from build123d import *

# Parameters (mm, degrees)
F0_R     = 33
F1_DEPTH = 10
F2_R     = 31.5
F3_DEPTH = 8
F5_DEPTH = 1
F6_R     = 1


with BuildPart() as f1:
    # F0 (on Top) → F1 (new body)
    with BuildSketch(Plane.XY):
        Circle(F0_R)
    extrude(amount=F1_DEPTH)

    # F2 (on face) → F3 (cut)
    with BuildSketch(Plane(origin=(0, 0, 0), x_dir=(1, 0, 0), z_dir=(0, 0, -1))):
        Circle(F2_R)
    extrude(amount=-F3_DEPTH, mode=Mode.SUBTRACT)

    # F4 (on face) → F5 (join)
    with BuildSketch(Plane(origin=(0, 0, 0), x_dir=(1, 0, 0), z_dir=(0, 0, -1))):
        with BuildLine():
            Line((16.1904761905, 25.2560582975), (17, 26.5188612124))
            ThreePointArc((17, 26.5188612124), (0, 31.5), (-17, 26.5188612124))
            Line((-17, 26.5188612124), (-16.1904761905, 25.2560582975))
            ThreePointArc((-16.1904761905, 25.2560582975), (0, 30), (16.1904761905, 25.2560582975))
        make_face()
        with BuildLine():
            Line((-29.9676261803, 1.3933345316), (-31.4660074893, 1.4630012582))
            ThreePointArc((-31.4660074893, 1.4630012582), (-27.2798002192, -15.75), (-14.4660074893, -27.9818624705))
            Line((-14.4660074893, -27.9818624705), (-13.7771499898, -26.6493928291))
            ThreePointArc((-13.7771499898, -26.6493928291), (-25.9807621135, -15), (-29.9676261803, 1.3933345316))
        make_face()
        with BuildLine():
            Line((13.7771499898, -26.6493928291), (14.4660074893, -27.9818624705))
            ThreePointArc((14.4660074893, -27.9818624705), (27.2798002192, -15.75), (31.4660074893, 1.4630012582))
            Line((31.4660074893, 1.4630012582), (29.9676261803, 1.3933345316))
            ThreePointArc((29.9676261803, 1.3933345316), (25.9807621135, -15), (13.7771499898, -26.6493928291))
        make_face()
    extrude(amount=-F5_DEPTH)

    # F6
    f6_edges = [f1.edges().sort_by_distance(p)[0] for p in [
        (29.967626, -1.393335, 0.5),
        (13.77715, 26.649393, 0.5),
        (16.190476, -25.256058, 0.5),
        (-13.77715, 26.649393, 0.5),
        (-29.967626, -1.393335, 0.5),
        (-16.190476, -25.256058, 0.5),
    ]]
    fillet(f6_edges, radius=F6_R)


solid = f1.part
Could you check a few things on this model? Use its own coordinates, in mm. A direction names the side the tool comes from. Coordinates: 2 decimals unless noted, no trailing zeros. Write each loop counter-clockwise with the first axis right and the second up, starting at its lowest first coordinate (ties: lowest second). Pieces come first, ordered by that corner, then holes. Notation, with made-up numbers: M 22,-13.5 L 59,-13.5 A11 ccw 59,3.5 Z; hole C -8,17 d8. An arc over 180 degrees is marked long. One line per question, with ' | ' between items.
1) If we mould it in two halves opening along Z, with no side actions, what happens to faces 4 (the face through (29.1, 12.06, 3.94)), 5 (the face through (15, 27, 0)), 6 (the face through (0, 0, 10))? For each: released by +Z, released by -Z, zero draft, split by the parting line, or undercut.
Checks:
face 4: undercut | face 5: released by -Z | face 6: released by +Z
2) Imagine slicing it at A-A, the plane x = 0. Write out the boundary of the cut face in (y, z), and give its area (4 significant figures).
Checks:
outline: M -33,0 L -30,0 L -30,1 L -31.5,1 L -31.5,8 L 31.5,8 L 31.5,0 L 33,0 L 33,10 L -33,10 Z | area: 157.5 mm²
3) Imagine slicing it at B-B, the plane z = 6. Write out the boundary of the cut face in (x, y), and give its area (3 significant figures).
Checks:
outline: C 0,0 d66; hole C 0,0 d63 | area: 304 mm²
4) Imagine slicing it at D-D, the plane x = -25.5. Write out the boundary of the cut face in (y, z), and give its area (3 significant figures).
Checks:
outline: M -20.95,0 L -18.49,0 L -18.49,8 L 18.49,8 L 18.49,1 L 15.8,1 L 15.8,0 L 20.95,0 L 20.95,10 L -20.95,10 Z | area: 126 mm²
5) For pin 1 Ø3 at (x, y) = (2.5, 13) entering from -Z; pin 2 Ø3 at (y, z) = (11, 7.5) entering from -X; pin 3 Ø5 at (y, z) = (-4.5, 8) entering from -X, each with a flat end and sliding along its axis, tell me the tip position at first contact or that it passes through.
Checks:
pin 1: z = 8 | pin 2: x = -31.6 | pin 3: x = -32.94
6) Imagine slicing it at C-C, the plane y = -22. Write out the boundary of the cut face in (x, z), and give its area (3 significant figures).
Checks:
outline: M -24.6,0 L -22.54,0 L -22.54,8 L 22.54,8 L 22.54,0 L 24.6,0 L 24.6,10 L -24.6,10 Z | area: 131 mm²
7) I need wall thicknesses on probe 1 along Y at (x, z) = (0, 3.5); probe 2 along Z at (x, y) = (-11, -19); probe 3 along Y at (x, z) = (22.5, 4.5). Which ranges of each line are inside material? Lowest first, please. Write a range as [from, to].
Checks:
probe 1: [-33, -31.5], [31.5, 33] | probe 2: [8, 10] | probe 3: [-24.14, -22.05], [22.05, 24.14]
8) For faces 1 (the face through (30.5, -12.6, 4.9)), 2 (the face through (26.093, 14.804, 0.493)), 3 (the face through (-26.1, 15.4, 1)), which set-ups out of +Z, -Z, +X, -X, +Y, -Y let a thin tool reach every point of the face, with its end or its side?
Checks:
face 1: +Z, -Z | face 2: -Z | face 3: none
